Can you work these out from the drawing? Everything is in mm from the part's minimum corner. Coordinates: 2 decimals unless noted, no trailing zeros. Loops run counter-clockwise (first coordinate to the right, second up) from the corner with the lowest first, then second, coordinate; pieces in that order, holes last.
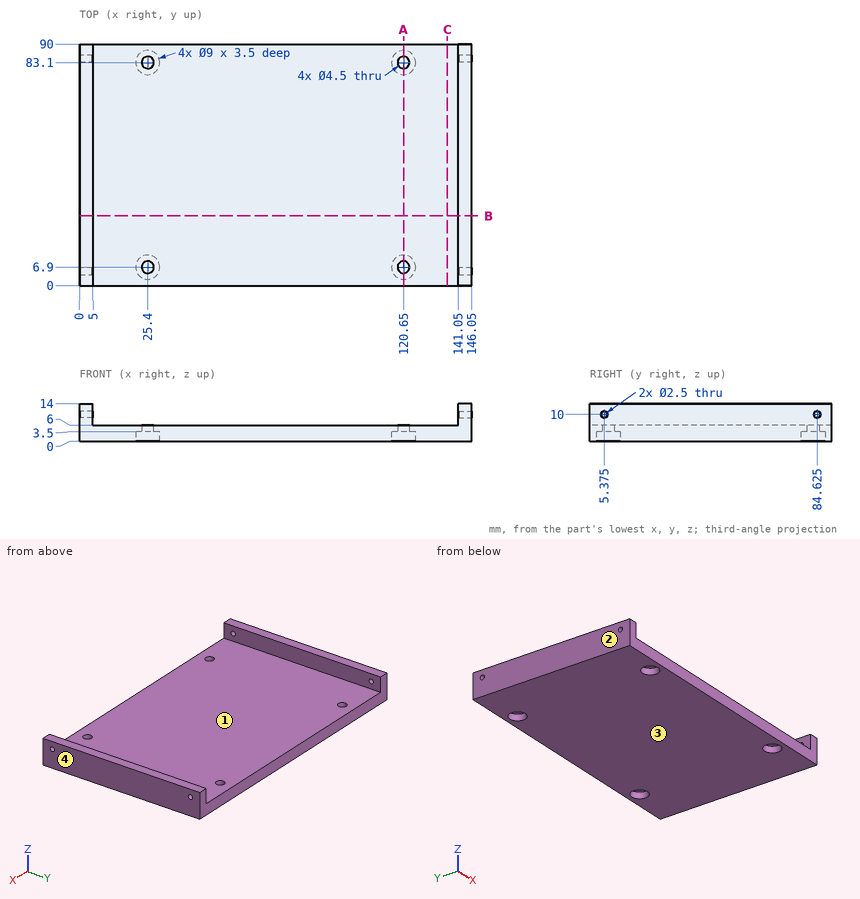
Item 1: We'd pull the mould along X, two halves only. Please class the marked faces 1, 2, 3 and 4: +X half, -X half, draft (parallel to the pull), parting line (faces both ways), or undercut.
Results are:
face 1: undercut
face 2: -X half
face 3: draft
face 4: +X half
Item 2: Suppose I cut it at A-A, the plane x = 120.65. Please give me the cut outline in (y, z), plus the area to 4 significant figures.
Results are:
outline: (0, 0) - (2.4, 0) - (2.4, 3.5) - (4.65, 3.5) - (4.65, 6) - (0, 6) - close; (9.15, 3.5) - (11.4, 3.5) - (11.4, 0) - (78.6, 0) - (78.6, 3.5) - (80.85, 3.5) - (80.85, 6) - (9.15, 6) - close; (85.35, 3.5) - (87.6, 3.5) - (87.6, 0) - (90, 0) - (90, 6) - (85.35, 6) - close
area: 454.5 mm2
Item 3: I'm going to push flat-ended pins straight in: P1, Ø7, axis at x = 120.65, y = 6.9, coming from the +Z side; P2, Ø5.5, axis at x = 120.65, y = 83.1, coming from the -Z side. Where does each tip first touch, or does it pass through?
Results are:
P1: stops at z = 6
P2: stops at z = 3.5
Item 4: Suppose I cut it at C-C, the plane x = 137. Please give me the cut outline in (y, z).
Results are:
outline: (0, 0) - (90, 0) - (90, 6) - (0, 6) - close
Item 5: Suppose I cut it at B-B, the plane y = 26. Please give me the cut outline in (x, z).
Results are:
outline: (0, 0) - (146.05, 0) - (146.05, 14) - (141.05, 14) - (141.05, 6) - (5, 6) - (5, 14) - (0, 14) - close
Item 6: I need wall thicknesses on line 1 along Y through (x, z) = (25.4, 1); line 2 along Y through (x, z) = (120.65, 4.95); line 3 along X through (y, z) = (6.9, 4.5). Which ranges of each line are inside material? Lowest first, please.
Results are:
line 1: y = 0 to 2.4, 11.4 to 78.6, 87.6 to 90
line 2: y = 0 to 4.65, 9.15 to 80.85, 85.35 to 90
line 3: x = 0 to 23.15, 27.65 to 118.4, 122.9 to 146.05
